Work out the finished part from the listing and answer in its coordinate system (mm). Face numbers are marked on the shaded views. Coordinates: 2 decimals unless noted, no trailing zeros. Write each loop counter-clockwise with the first axis right and the second up, starting at its lowest first coordinate (ties: lowest second). Pieces come first, ordered by that corner, then holes. Notation, with made-up numbers: M -16,55.5 L -5,55.5 A35 ccw -5,91.5 Z; hole C 3.5,30 d9. An arc over 180 degrees is marked long. Use CSV: the item, a comma, the result in double quotes.
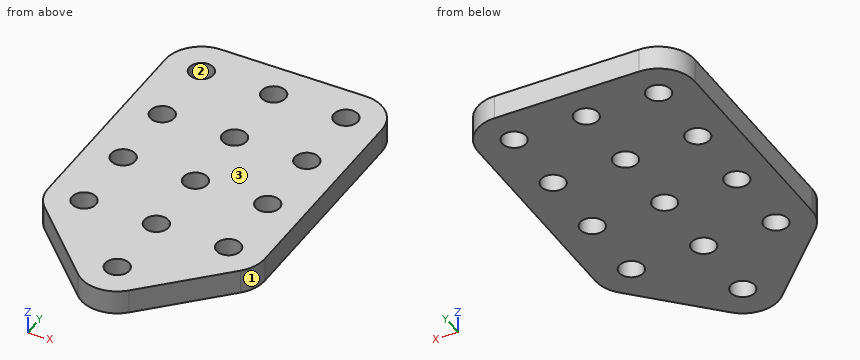
from build123d import *

# Parameters (mm, degrees)
MODEL_R                 = 1.5
SALIENTE_EXTRUIR1_DEPTH = 3


with BuildPart() as part:
    # Model → Saliente-Extruir1 (new body)
    with BuildSketch(Plane.XY):
        with BuildLine():
            Line((174.227054575, 213.178720063), (174.227054575, 204.178720063))
            ThreePointArc((174.227054575, 204.178720063), (174.569596678, 202.456644617), (175.545074059, 200.996739548))
            Line((175.545074059, 200.996739548), (184.545074059, 191.996739548))
            ThreePointArc((184.545074059, 191.996739548), (187.727054575, 190.678720063), (190.90903509, 191.996739548))
            Line((190.90903509, 191.996739548), (199.90903509, 200.996739548))
            ThreePointArc((199.90903509, 200.996739548), (200.884512471, 202.456644617), (201.227054575, 204.178720063))
            Line((201.227054575, 204.178720063), (201.227054575, 231.178720063))
            ThreePointArc((201.227054575, 231.178720063), (199.90903509, 234.360700578), (196.727054575, 235.678720063))
            Line((196.727054575, 235.678720063), (178.727054575, 235.678720063))
            ThreePointArc((178.727054575, 235.678720063), (175.545074059, 234.360700578), (174.227054575, 231.178720063))
            Line((174.227054575, 231.178720063), (174.227054575, 213.178720063))
        make_face()
        with Locations((187.727054575, 204.178720063)):
            Circle(MODEL_R, mode=Mode.SUBTRACT)
        with Locations((178.727054575, 204.178720063)):
            Circle(MODEL_R, mode=Mode.SUBTRACT)
        with Locations((187.727054575, 213.178720063)):
            Circle(MODEL_R, mode=Mode.SUBTRACT)
        with Locations((178.727054575, 213.178720063)):
            Circle(MODEL_R, mode=Mode.SUBTRACT)
        with Locations((196.727054575, 213.178720063)):
            Circle(MODEL_R, mode=Mode.SUBTRACT)
        with Locations((187.727054575, 195.178720063)):
            Circle(MODEL_R, mode=Mode.SUBTRACT)
        with Locations((196.727054575, 204.178720063)):
            Circle(MODEL_R, mode=Mode.SUBTRACT)
        with Locations((187.727054575, 222.178720063)):
            Circle(MODEL_R, mode=Mode.SUBTRACT)
        with Locations((178.727054575, 222.178720063)):
            Circle(MODEL_R, mode=Mode.SUBTRACT)
        with Locations((196.727054575, 222.178720063)):
            Circle(MODEL_R, mode=Mode.SUBTRACT)
        with Locations((187.727054575, 231.178720063)):
            Circle(MODEL_R, mode=Mode.SUBTRACT)
        with Locations((178.727054575, 231.178720063)):
            Circle(MODEL_R, mode=Mode.SUBTRACT)
        with Locations((196.727054575, 231.178720063)):
            Circle(MODEL_R, mode=Mode.SUBTRACT)
    extrude(amount=SALIENTE_EXTRUIR1_DEPTH)


solid = part.part
Item 1: The part is cut by section D-D (y = 199). Write down the section's boundary in (x, z), then the cut area to 3 significant figures.
Answer:
outline,"M 177.54,0 L 197.91,0 L 197.91,3 L 177.54,3 Z"
area,"61.1 mm2"
Item 2: Consider probe 1 along X at (y, z) = (205.5, 2.55); probe 2 along X at (y, z) = (212, 2); probe 3 along Y at (x, z) = (197, 1). Determine where each line is inside the solid, lowest interval first.
Answer:
probe 1,"x = 174.23 to 178.02, 179.44 to 187.02, 188.44 to 196.02, 197.44 to 201.23"
probe 2,"x = 174.23 to 177.8, 179.65 to 186.8, 188.65 to 195.8, 197.65 to 201.23"
probe 3,"y = 198.09 to 202.7, 205.65 to 211.7, 214.65 to 220.7, 223.65 to 229.7, 232.65 to 235.67"
Item 3: Given pin 1 (2.5 mm diameter, centred on x = 187.73, y = 195.18, fed in from +Z); pin 2 (1 mm diameter, centred on x = 177, z = 1, fed in from +Y), each flat-ended and moving along its own axis, determine where each tip first touches the part or whether it passes through.
Answer:
pin 1,"passes through"
pin 2,"stops at y = 235.51"
Item 4: The part is cut by section B-B (z = 2.4). Count the separate pieces of the cut face and the enclosed holes in it, then the cut area to 3 significant figures.
Answer:
separate pieces,"1"
enclosed holes,"13"
area,"977 mm2"
Item 5: The part is cut by section A-A (y = 205). Write down the section's boundary in (x, z), then the cut area to 3 significant figures.
Answer:
outline,"M 174.23,0 L 177.47,0 L 177.47,3 L 174.23,3 Z; M 179.98,0 L 186.47,0 L 186.47,3 L 179.98,3 Z; M 188.98,0 L 195.47,0 L 195.47,3 L 188.98,3 Z; M 197.98,0 L 201.23,0 L 201.23,3 L 197.98,3 Z"
area,"58.4 mm2"
Item 6: For a pull along X with two mould halves and no side action, classify the marked faces 1, 2 and 3 as released by +X, released by -X, zero draft, split by the parting line, or undercut.
Answer:
face 1,"released by +X"
face 2,"undercut"
face 3,"zero draft"
Item 7: The part is cut by section C-C (x = 191.75). Write down the section's boundary in (y, z), then the cut area to 3 significant figures.
Answer:
outline,"M 192.84,0 L 235.68,0 L 235.68,3 L 192.84,3 Z"
area,"129 mm2"
